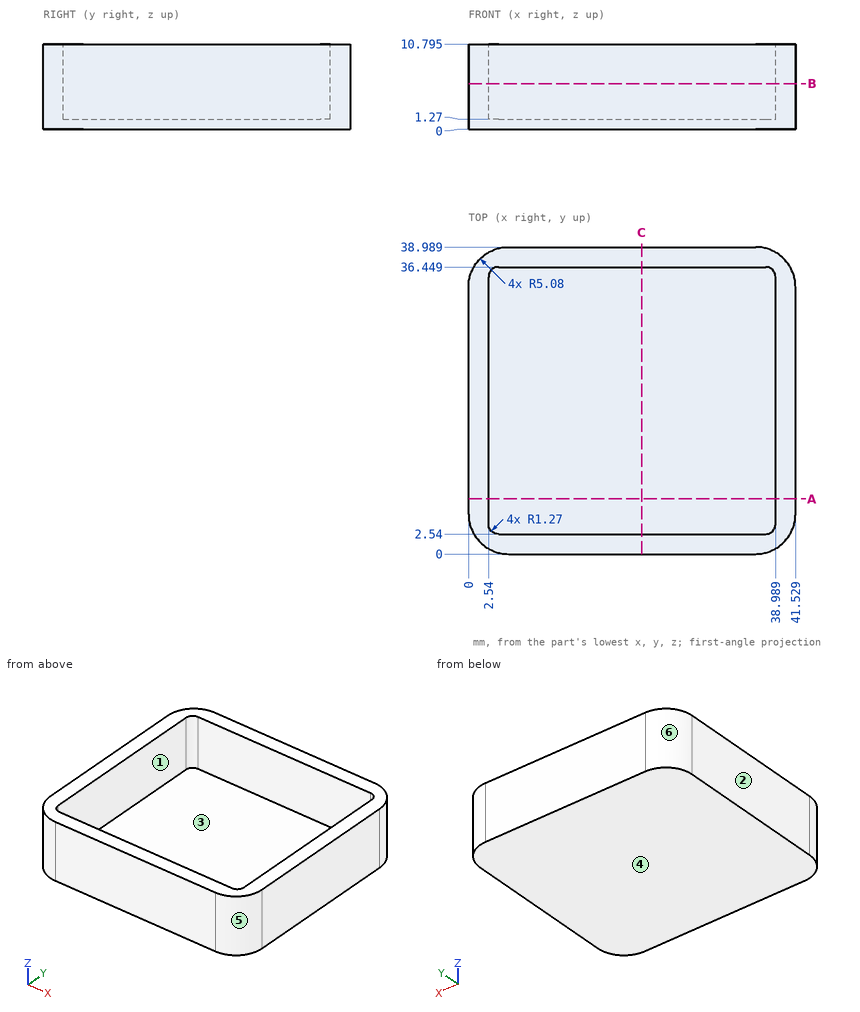
Study the drawing (mm; zero at the part's minimum x, y, z) and answer. A direction names the side the tool comes from. Coordinates: 2 decimals unless noted, no trailing zeros. Write each loop counter-clockwise with the first axis right and the second up, starting at its lowest first coordinate (ties: lowest second). Pieces come first, ordered by that corner, then holes. Notation, with made-up numbers: (-34, -14.5) - (18, -14.5) arc R21 ccw to (18, 6.5) - close; hole circle Ø9 at (70, 2). An arc over 180 degrees is marked (long way). Return JSON: item names as keys, results as strings. Group by question number.
1. Determine the mould class of the marked faces 3, 4, 5 and 6 for opening direction Y: released by +Y, released by -Y, zero draft, split by the parting line, or undercut.
2. Straight lines are drawn through the part: L1, parallel to Y at x = 32, z = 3; L2, parallel to X at y = 20, z = 6; L3, parallel to Z at x = 27, y = 18. For each, find the intervals that lie inside material, in ascending order.
3. A cutting plane is placed at A-A, the plane y = 7. Determine the outline of the cut face in (x, z) (3 decimals), plus the area to 3 significant figures.
4. A cutting plane is placed at C-C, the plane x = 22. Determine the outline of the cut face in (y, z) (3 decimals).
5. Given pin 1 (10 mm diameter, centred on x = 32.5, y = 9.5, fed in from +Z); pin 2 (3 mm diameter, centred on x = 12, y = 34, fed in from -Z), each flat-ended and moving along its own axis, determine where each tip first touches the part or whether it passes through.
6. Which of the six approach directions +Z, -Z, +X, -X, +Y, -Y give full straight-line access (tool end or side, diameter ignored) to the marked faces 1 and 2?
7. A cutting plane is placed at B-B, the plane z = 5.75. Determine the outline of the cut face in (x, y).
Ans:
{
 "1": {"face 3": "undercut", "face 4": "zero draft", "face 5": "released by -Y", "face 6": "released by +Y"},
 "2": {"L1": "0 to 2.54, 36.45 to 38.99", "L2": "0 to 2.54, 38.99 to 41.53", "L3": "0 to 1.27"},
 "3": {"outline": "(0, 0) - (41.529, 0) - (41.529, 10.795) - (38.989, 10.795) - (38.989, 1.27) - (2.54, 1.27) - (2.54, 10.795) - (0, 10.795) - close", "area": "101 mm²"},
 "4": {"outline": "(0, 0) - (38.989, 0) - (38.989, 10.795) - (36.449, 10.795) - (36.449, 1.27) - (2.54, 1.27) - (2.54, 10.795) - (0, 10.795) - close"},
 "5": {"pin 1": "z = 1.27", "pin 2": "z = 0"},
 "6": {"face 1": "+Z", "face 2": "+Z, -Z, -X, +Y, -Y"},
 "7": {"outline": "(0, 5.08) arc R5.08 ccw to (5.08, 0) - (36.45, 0) arc R5.08 ccw to (41.53, 5.08) - (41.53, 33.91) arc R5.08 ccw to (36.45, 38.99) - (5.08, 38.99) arc R5.08 ccw to (0, 33.91) - close; hole (2.54, 3.81) arc R1.27 ccw to (3.81, 2.54) - (37.72, 2.54) arc R1.27 ccw to (38.99, 3.81) - (38.99, 35.18) arc R1.27 ccw to (37.72, 36.45) - (3.81, 36.45) arc R1.27 ccw to (2.54, 35.18) - close"}
}
